from build123d import *

# Parameters (mm, degrees)
SKETCH1_W           = 152.4
SKETCH1_H           = 304.8
BOSS_EXTRUDE1_DEPTH = 1.5875
SKETCH3_R           = 2.6543
SKETCH3_R_2         = 3.3782
CUT_EXTRUDE1_DEPTH  = 4.175
FILLET1_R           = 7.62
CUT_EXTRUDE2_START  = -4.175
CUT_EXTRUDE2_DEPTH  = 5.175
CUT_EXTRUDE3_DEPTH  = 4.175
CUT_EXTRUDE4_DEPTH  = 4.175


with BuildPart() as part:
    # Sketch1 → Boss-Extrude1 (new body, symmetric)
    with BuildSketch(Plane(origin=(0, 0, 0), x_dir=(1, 0, 0), z_dir=(0, 1, 0))):
        Rectangle(SKETCH1_W, SKETCH1_H)
    extrude(amount=BOSS_EXTRUDE1_DEPTH, both=True)

    # Sketch3 → Cut-Extrude1 (cut, through all)
    with BuildSketch(Plane(origin=(0, 1.5875, 0), x_dir=(1, 0, 0), z_dir=(0, 1, 0))):
        with Locations((45.72, -109.22)):
            Circle(SKETCH3_R)
        with Locations((45.72, 26.67)):
            Circle(SKETCH3_R)
        with Locations((64.008, 132.08)):
            Circle(SKETCH3_R_2)
        with Locations((64.008, -132.08)):
            Circle(SKETCH3_R_2)
    cut_extrude1 = extrude(amount=-CUT_EXTRUDE1_DEPTH, mode=Mode.SUBTRACT)

    # Mirror1: Cut-Extrude1 across plane
    add(cut_extrude1.mirror(Plane(origin=(0, 0, 0), x_dir=(0, 0, 1), z_dir=(1, 0, 0))), mode=Mode.SUBTRACT)

    # Fillet1
    fillet1_edges = [part.edges().sort_by_distance(p)[0] for p in [
        (76.2, 0, 152.4),
        (-76.2, 0, 152.4),
        (-76.2, 0, -152.4),
        (76.2, 0, -152.4),
    ]]
    fillet(fillet1_edges, radius=FILLET1_R)

    # Sketch4 → Cut-Extrude2 (cut)
    with BuildSketch(Plane(origin=(0, 1.5875, 0), x_dir=(1, 0, 0), z_dir=(0, 1, 0)).offset(CUT_EXTRUDE2_START)):
        with BuildLine():
            Line((-753.455657881, 152.4), (-68.58, 152.4))
            Line((-68.58, 152.4), (-37.674288314, 152.4))
            ThreePointArc((-37.674288314, 152.4), (-29.15486932, 149.796340451), (-23.546430197, 142.875))
            ThreePointArc((-23.546430197, 142.875), (0, 127), (23.546430197, 142.875))
            ThreePointArc((23.546430197, 142.875), (29.15486932, 149.796340451), (37.674288314, 152.4))
            Line((37.674288314, 152.4), (68.58, 152.4))
            Line((68.58, 152.4), (753.455657881, 152.4))
            Line((753.455657881, 152.4), (753.455657881, 1522.151315762))
            Line((753.455657881, 1522.151315762), (-753.455657881, 1522.151315762))
            Line((-753.455657881, 1522.151315762), (-753.455657881, 152.4))
        make_face()
    cut_extrude2 = extrude(amount=CUT_EXTRUDE2_DEPTH, mode=Mode.SUBTRACT)

    # Mirror2: Cut-Extrude2 across plane
    add(cut_extrude2.mirror(Plane.XY), mode=Mode.SUBTRACT)

    # Sketch7 → Cut-Extrude3 (cut, through all)
    with BuildSketch(Plane(origin=(0, 1.5875, 0), x_dir=(1, 0, 0), z_dir=(0, 1, 0))):
        with BuildLine():
            Line((65.518901805, 109.877508821), (65.518901805, 42.4057621))
            ThreePointArc((65.518901805, 42.4057621), (60.96, 37.846860295), (56.401098195, 42.4057621))
            Line((56.401098195, 42.4057621), (56.401098195, 109.877508821))
            ThreePointArc((56.401098195, 109.877508821), (60.96, 114.436410627), (65.518901805, 109.877508821))
        make_face()
        with BuildLine():
            Line((65.518901805, 1.973635461), (65.518901805, -90.990364539))
            ThreePointArc((65.518901805, -90.990364539), (60.96, -95.549266345), (56.401098195, -90.990364539))
            Line((56.401098195, -90.990364539), (56.401098195, 1.973635461))
            ThreePointArc((56.401098195, 1.973635461), (60.96, 6.532537266), (65.518901805, 1.973635461))
        make_face()
    cut_extrude3 = extrude(amount=-CUT_EXTRUDE3_DEPTH, mode=Mode.SUBTRACT)

    # Mirror3: Cut-Extrude3 across plane
    add(cut_extrude3.mirror(Plane(origin=(0, 0, 0), x_dir=(0, 0, 1), z_dir=(1, 0, 0))), mode=Mode.SUBTRACT)

    # Sketch9 → Cut-Extrude4 (cut, through all)
    with BuildSketch(Plane.XZ.offset(1.5875)):
        with BuildLine():
            Line((-14.5923, -61.722), (-14.5923, -103.398249639))
            ThreePointArc((-14.5923, -103.398249639), (-13.42547703, -106.718929839), (-10.437940285, -108.579848169))
            ThreePointArc((-10.437940285, -108.579848169), (37.40844001, -91.808826826), (43.529723769, -41.479181989))
            ThreePointArc((43.529723769, -41.479181989), (40.754786716, -33.137895831), (43.391609306, -24.751925581))
            Line((43.391609306, -24.751925581), (47.393812046, -19.116690889))
            ThreePointArc((47.393812046, -19.116690889), (48.123241377, -17.656049777), (48.3743, -16.042820352))
            Line((48.3743, -16.042820352), (48.3743, 99.374229362))
            ThreePointArc((48.3743, 99.374229362), (47.460552946, 102.351896493), (45.03387068, 104.304496914))
            Line((45.03387068, 104.304496914), (21.617623949, 113.6523))
            Line((21.617623949, 113.6523), (-21.617623949, 113.6523))
            Line((-21.617623949, 113.6523), (-45.03387068, 104.304496914))
            ThreePointArc((-45.03387068, 104.304496914), (-47.460552946, 102.351896493), (-48.3743, 99.374229362))
            Line((-48.3743, 99.374229362), (-48.3743, -19.388666667))
            ThreePointArc((-48.3743, -19.388666667), (-47.630351224, -21.184717891), (-45.8343, -21.928666667))
            Line((-45.8343, -21.928666667), (-36.576, -21.928666667))
            ThreePointArc((-36.576, -21.928666667), (-34.779948776, -22.672615442), (-34.036, -24.468666667))
            Line((-34.036, -24.468666667), (-34.036, -32.088666667))
            ThreePointArc((-34.036, -32.088666667), (-33.292051224, -33.884717891), (-31.496, -34.628666667))
            Line((-31.496, -34.628666667), (-5.08, -34.628666667))
            ThreePointArc((-5.08, -34.628666667), (-3.283948776, -35.372615442), (-2.54, -37.168666667))
            Line((-2.54, -37.168666667), (-2.54, -45.360175429))
            ThreePointArc((-2.54, -45.360175429), (-3.034932492, -46.866594656), (-4.326849518, -47.785946307))
            ThreePointArc((-4.326849518, -47.785946307), (-11.748912833, -53.06762154), (-14.5923, -61.722))
        make_face()
    extrude(amount=-CUT_EXTRUDE4_DEPTH, mode=Mode.SUBTRACT)


solid = part.part
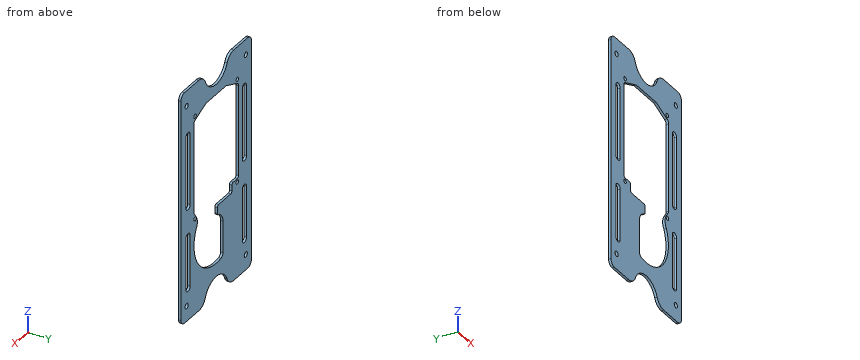
CAD build for the part. Positions are in the model's coordinates, mm. Round coordinates to 2 decimals unless told otherwise and drop trailing zeros. Write each loop counter-clockwise with the first axis right and the second up, starting at its lowest first coordinate (ties: lowest second). Pieces come first, ordered by that corner, then holes.
(1) Slice it at C-C, the plane x = 33. Write the cut outline in (y, z).
(2) Drop a flat-ended pin along its axis: P1, Ø4, axis at x = 64.008, z = 132.08, coming from the -Y side. Give the stop position or say it passes through.
(3) Slice it at D-D, the plane z = -85.5. Write the cut outline in (x, y), and give its area (3 significant figures).
(4) Slice it at B-B, the plane y = -0.75. Count the separate pieces of the cut face and the enclosed holes in it, and give its area (3 significant figures).
(5) Slice it at A-A, the plane z = 132.08. Write the cut outline in (x, y).
(6) Probe line 1 along X through (y, z) = (1.1, 73); line 2 along X through (y, z) = (-0.2, -3.5); line 3 along X through (y, z) = (0.8, -8). List the from-to ranges inside material, lowest first.
From the geometry:
1. outline: (-1.59, -151.67) - (1.59, -151.67) - (1.59, -96.59) - (-1.59, -96.59) - close; (-1.59, 109.11) - (1.59, 109.11) - (1.59, 151.67) - (-1.59, 151.67) - close
2. P1: passes through
3. outline: (-76.2, -1.59) - (-65.52, -1.59) - (-65.52, 1.59) - (-76.2, 1.59) - close; (-56.4, -1.59) - (-14.59, -1.59) - (-14.59, 1.59) - (-56.4, 1.59) - close; (41.7, -1.59) - (56.4, -1.59) - (56.4, 1.59) - (41.7, 1.59) - close; (65.52, -1.59) - (76.2, -1.59) - (76.2, 1.59) - (65.52, 1.59) - close
3. area: 247 mm2
4. separate pieces: 1
4. enclosed holes: 13
4. area: 23,100 mm2
5. outline: (-76.2, -1.59) - (-67.39, -1.59) - (-67.39, 1.59) - (-76.2, 1.59) - close; (-60.63, -1.59) - (-15.24, -1.59) - (-15.24, 1.59) - (-60.63, 1.59) - close; (15.24, -1.59) - (60.63, -1.59) - (60.63, 1.59) - (15.24, 1.59) - close; (67.39, -1.59) - (76.2, -1.59) - (76.2, 1.59) - (67.39, 1.59) - close
6. line 1: x = -76.2 to -65.52, -56.4 to -48.37, 48.37 to 56.4, 65.52 to 76.2
6. line 2: x = -76.2 to -65.26, -56.66 to -48.37, 48.37 to 56.66, 65.26 to 76.2
6. line 3: x = -76.2 to -48.37, 48.37 to 76.2
